Geometry: final body of the model. Coordinates: model frame, mm. Face numbers are marked on the shaded views. A direction names the side the tool comes from. Give positions to 0.01 mm unless a question says otherwise; leave off trailing zeros. Order: outer loops, then holes, each group sorted by start corner. A loop starts at its lowest first (then second) coordinate and runs counter-clockwise, first axis right, second up. Notation, with made-up numbers: (-14.5, -5.75) - (30.5, -5.75) arc R36 cw to (30.5, 33.25) - close; hole circle Ø8 at (11.25, 75). An arc over 180 degrees is marked (long way). Use one line per item in the form item = value.
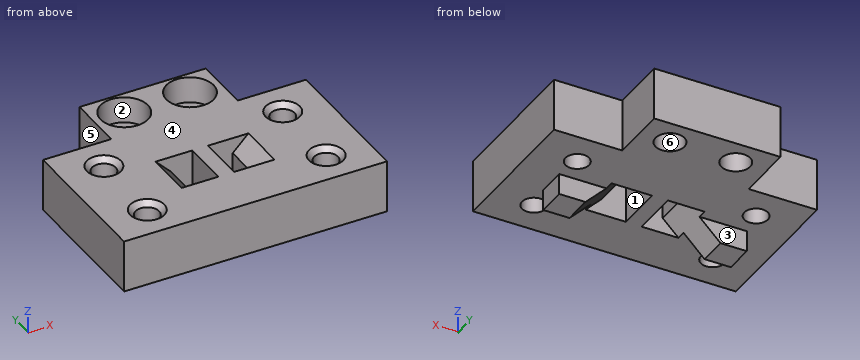
from build123d import *

# Parameters (mm, degrees)
PAD_DEPTH        = 10
HOLE_D           = 5.5
HOLE_CBORE_D     = 9
HOLE_CBORE_DEPTH = 5
POCKET_DEPTH     = 9
SKETCH004_R      = 2.25
HOLE001_DEPTH    = 10.001
CHAMFER_SIZE     = 1
PAD001_DEPTH     = 2.75


with BuildPart() as part:
    # Sketch → Pad (new body)
    with BuildSketch(Plane.XY):
        Polygon((0, 0), (24, 0), (24, -11), (37, -11), (37, -39), (-13, -39), (-13, -11), (0, -11), align=None)
    extrude(amount=PAD_DEPTH)

    # Hole (through all)
    with Locations(Plane.XY.offset(10)):
        with Locations((5.75, -5), (18.25, -5)):
            CounterBoreHole(HOLE_D / 2, HOLE_CBORE_D / 2, HOLE_CBORE_DEPTH)

    # Sketch003 (on Face6 of Hole) → Pocket (cut)
    with BuildSketch(Plane(origin=(0, -20.5, 0), x_dir=(-1, 0, 0), z_dir=(0, 1, 0))):
        Polygon((-3.163025, 0), (-6.163025, 3), (-6.163025, 7), (-3.163025, 10), (-10.163025, 10), (-10.163025, 0), align=None)
        Polygon((-20.836975, 10), (-13.163025, 10), (-13.163025, 0), (-20.836975, 0), (-17.836975, 3), (-17.836975, 7), align=None)
    extrude(amount=-POCKET_DEPTH, mode=Mode.SUBTRACT)

    # Sketch004 (on Face5 of Pocket) → Hole001 (cut, through all)
    with BuildSketch(Plane.XY.offset(10)):
        with Locations((-5, -17.5)):
            Circle(SKETCH004_R)
        with Locations((-5, -32.5)):
            Circle(SKETCH004_R)
        with Locations((29, -32.5)):
            Circle(SKETCH004_R)
        with Locations((29, -17.5)):
            Circle(SKETCH004_R)
    extrude(amount=-HOLE001_DEPTH, mode=Mode.SUBTRACT)

    # Chamfer
    chamfer_edges = [part.edges().sort_by_distance(p)[0] for p in [
        (-7.25, -17.5, 10),
        (-7.25, -32.5, 10),
        (26.75, -17.5, 10),
        (26.75, -32.5, 10),
    ]]
    chamfer(chamfer_edges, length=CHAMFER_SIZE)

    # Sketch005 → Pad001 (join, symmetric)
    with BuildSketch(Plane.XZ.offset(25)):
        Polygon((-0.836975, -4), (-5.836975, -4), (-5.836975, 0), (3.163025, 0), align=None)
        Polygon((20.836975, 0), (24.836975, -4), (29.836975, -4), (29.836975, 0), align=None)
    extrude(amount=PAD001_DEPTH, both=True)


solid = part.part
(1) Pull-direction query (X, two-part tool) for the marked faces 4, 5 and 6; classes: released by +X, released by -X, zero draft, split by the parting line, or undercut.
Computed values:
face_4 = zero draft
face_5 = released by -X
face_6 = undercut
(2) Ray query, line 1 along Y through (x, z) = (29, 2.75); line 2 along X through (y, z) = (-28, 3); line 3 along Y through (x, z) = (5.75, 1.55). Return the intervals inside material, ascending.
Computed values:
line_1 = -39 to -34.75, -30.25 to -19.75, -15.25 to -11
line_2 = -13 to 6.16, 10.16 to 13.16, 17.84 to 37
line_3 = -39 to -29.5, -20.5 to -7.75, -2.25 to 0
(3) Cut plane D-D on z = -2.75. Output: boundary loops of the cut face in (x, y).
Computed values:
outline = (-5.84, -27.75) - (0.41, -27.75) - (0.41, -22.25) - (-5.84, -22.25) - close; (23.59, -27.75) - (29.84, -27.75) - (29.84, -22.25) - (23.59, -22.25) - close
(4) Contact query for flat-ended pins moving along their axis: pin 1 Ø3 at (x, z) = (-3.5, 4) entering from +Y; pin 2 Ø1.2 at (x, z) = (25, -3) entering from -Y; pin 3 Ø8 at (y, z) = (-6, 6.5) entering from -X. Output: stop coordinate, or through.
Computed values:
pin_1 = -11
pin_2 = -27.75
pin_3 = 0
(5) Reachability of the marked faces 1, 2 and 3 from +Z, -Z, +X, -X, +Y, -Y: full face, straight path, thin tool, end or side. Return the list, or none.
Computed values:
face_1 = +Z, -Z
face_2 = +Z
face_3 = -Z, +X, -X, +Y
(6) Cut plane B-B on x = -5. Output: boundary loops of the cut face in (y, z), plus the area to 3 significant figures.
Computed values:
outline = (-39, 0) - (-34.75, 0) - (-34.75, 9) - (-35.75, 10) - (-39, 10) - close; (-30.25, 0) - (-27.75, 0) - (-27.75, -4) - (-22.25, -4) - (-22.25, 0) - (-19.75, 0) - (-19.75, 9) - (-20.75, 10) - (-29.25, 10) - (-30.25, 9) - close; (-15.25, 0) - (-11, 0) - (-11, 10) - (-14.25, 10) - (-15.25, 9) - close
area = 210 mm²
(7) Cut plane A-A on y = -17.5. Output: boundary loops of the cut face in (x, z).
Computed values:
outline = (-13, 0) - (-7.25, 0) - (-7.25, 9) - (-8.25, 10) - (-13, 10) - close; (-2.75, 0) - (26.75, 0) - (26.75, 9) - (25.75, 10) - (-1.75, 10) - (-2.75, 9) - close; (31.25, 0) - (37, 0) - (37, 10) - (32.25, 10) - (31.25, 9) - close
(8) Cut plane C-C on z = 5.75. Give the number of separate pieces and of enclosed holes in the cut face, plus the area to 3 significant figures.
Computed values:
separate_pieces = 1
enclosed_holes = 8
area = 1,400 mm²
